For this review, take the finished solid that the model builds, in its own axes (mm). A direction names the side the tool comes from. Coordinates: 2 decimals unless noted, no trailing zeros. Loops run counter-clockwise (first coordinate to the right, second up) from the corner with the lowest first, then second, coordinate; pieces in that order, holes last. Notation, with made-up numbers: (69, 37.25) -> (117, 37.25) arc R15 ccw to (117, 52.25) -> close; hole circle Ø8 at (84, 11.5). An arc over 180 degrees is marked (long way). Answer in a Markdown table with one row per item.
from build123d import *

# Parameters (mm, degrees)
BASES_W                              = 20.16
BASES_H                              = 40
BASE_DEPTH                           = 10
SHAFTHOLES_R                         = 3
SHAFT_HOLE_DEPTH                     = 25.527666012
MOUNTINGTABS_W                       = 19
MOUNTINGTABS_H                       = 2.4
MOUNTING_TAB_DEPTH                   = 7.2
MOUNTING_HOLE_DEPTH                  = 30.986770416
BOTTOMALIGNHOLES_R                   = 0.7
BOTTOM_ALIGN_HOLE_DEPTH              = 0.5
TRIANGULAR_TAB_DEPTH                 = 0.9
MOUNTING_TAB_FEATURES_M_COPY_1_DEPTH = 30.986770416
BORDERCUTS_W                         = 20.16
BORDERCUTS_H                         = 40
BORDERCUTS_W_2                       = 19.56
BORDERCUTS_H_2                       = 39.4
BORDER_CUT_DEPTH                     = 0.5
BORDER_CUT_F_R                       = 0.75
SHELL3_OUTLINE_W                     = 17.96
SHELL3_OUTLINE_H                     = 37.8
SHELL3_OUTLINE_R                     = 3.8
SHELL3_DEPTH                         = 9.2
SHELL3_2_OUTLINE_W                   = 18.56
SHELL3_2_OUTLINE_H                   = 38.4
SHELL3_2_OUTLINE_W_2                 = 17.96
SHELL3_2_OUTLINE_H_2                 = 37.8
SHELL3_2_DEPTH                       = 8.7
SHELL3_3_DEPTH                       = 1.6
SHELL3_START                         = 1.3
SHELL3_4_DEPTH                       = 0.3
SHELL3_START_2                       = 1.6
SHELL3_5_OUTLINE_W                   = 0.2
SHELL3_5_OUTLINE_H                   = 7.2
SHELL3_5_DEPTH                       = 0.083965765
SHELL3_START_3                       = -0.1
SHELL3_6_DEPTH                       = 0.2
SKETCH2_R                            = 4.5
CUT_EXTRUDE1_DEPTH                   = 3
SKETCH3_R                            = 6
SKETCH3_R_2                          = 5.5
BOSS_EXTRUDE1_DEPTH                  = 1.25
SKETCH3_4_R                          = 5.5
BOSS_EXTRUDE2_DEPTH                  = 1.5
SKETCH3_5_R                          = 5
BOSS_EXTRUDE3_DEPTH                  = 1.75
CUT_EXTRUDE7_DEPTH                   = 31.68299855
CUT_EXTRUDE7_DEPTH_BACK              = 31.68299855
SKETCH3_6_R                          = 3
BOSS_EXTRUDE4_DEPTH                  = 1
SKETCH6_R                            = 3
CUT_EXTRUDE8_DEPTH                   = 20
SKETCH7_W                            = 12.822327898
SKETCH7_H                            = 9.709392801
CUT_EXTRUDE9_DEPTH                   = 0.5
FILLET2_R                            = 0.3


with BuildPart() as part:
    # BaseS → BASE (new body)
    with BuildSketch(Plane(origin=(0, 0, 0), x_dir=(1, 0, 0), z_dir=(0, 1, 0))):
        Rectangle(BASES_W, BASES_H)
    extrude(amount=BASE_DEPTH)

    # ShaftHoleS → SHAFT HOLE (cut, through all)
    with BuildSketch(Plane(origin=(0, 10, 0), x_dir=(1, 0, 0), z_dir=(0, 1, 0))):
        with Locations(Location((0, 10, 0), (0, 0, 270))):
            Circle(SHAFTHOLES_R)
    extrude(amount=-SHAFT_HOLE_DEPTH, mode=Mode.SUBTRACT)

    # MountingTabS → MOUNTING TAB (add)
    with BuildSketch(Plane.XY.offset(20)):
        with Locations((0, 1.2)):
            Rectangle(MOUNTINGTABS_W, MOUNTINGTABS_H)
    mounting_tab = extrude(amount=MOUNTING_TAB_DEPTH)

    # MountingHoleS → MOUNTING HOLE (cut, through all)
    with BuildSketch(Plane(origin=(0, 2.4, 0), x_dir=(1, 0, 0), z_dir=(0, 1, 0))):
        with BuildLine():
            Line((-6.25, -26.6), (-6.25, -27.2))
            Line((-6.25, -27.2), (-3.75, -27.2))
            Line((-3.75, -27.2), (-3.75, -26.6))
            ThreePointArc((-3.75, -26.6), (-5, -22.479171307), (-6.25, -26.6))
        make_face()
    mounting_hole = extrude(amount=-MOUNTING_HOLE_DEPTH, mode=Mode.SUBTRACT)

    # MH M: MOUNTING HOLE across plane
    add(mounting_hole.mirror(Plane(origin=(0, 0, 0), x_dir=(0, 0, 1), z_dir=(1, 0, 0))), mode=Mode.SUBTRACT)

    # BottomAlignHoleS → BOTTOM ALIGN HOLE (cut)
    with BuildSketch(Plane.XZ):
        with Locations(Location((0, 25.2, 0), (0, 0, 270))):
            Circle(BOTTOMALIGNHOLES_R)
    bottom_align_hole = extrude(amount=-BOTTOM_ALIGN_HOLE_DEPTH, mode=Mode.SUBTRACT)

    # TriangularTabS → TRIANGULAR TAB (add, symmetric)
    with BuildSketch(Plane(origin=(0, 0, 0), x_dir=(0, 0, -1), z_dir=(1, 0, 0))):
        Polygon((-20, 2.4), (-27.2, 2.4), (-20, 3.2), align=None)
    triangular_tab = extrude(amount=TRIANGULAR_TAB_DEPTH, both=True)

    # MOUNTING TAB FEATURES M: MOUNTING TAB, MOUNTING HOLE, BOTTOM ALIGN HOLE, TRIANGULAR TAB across plane
    add(mounting_tab.mirror(Plane.XY))
    add(mounting_hole.mirror(Plane.XY), mode=Mode.SUBTRACT)
    add(bottom_align_hole.mirror(Plane.XY), mode=Mode.SUBTRACT)
    add(triangular_tab.mirror(Plane.XY))

    # MOUNTING TAB FEATURES M copy 1 sketch → MOUNTING TAB FEATURES M copy 1 (cut, through all)
    with BuildSketch(Plane(origin=(0, 2.4, 0), x_dir=(-1, 0, 0), z_dir=(0, 1, 0))):
        with BuildLine():
            Line((-6.25, -26.6), (-6.25, -27.2))
            Line((-6.25, -27.2), (-3.75, -27.2))
            Line((-3.75, -27.2), (-3.75, -26.6))
            ThreePointArc((-3.75, -26.6), (-5, -22.479171307), (-6.25, -26.6))
        make_face()
    extrude(amount=-MOUNTING_TAB_FEATURES_M_COPY_1_DEPTH, mode=Mode.SUBTRACT)

    # BorderCutS → BORDER CUT (cut)
    with BuildSketch(Plane(origin=(0, 10, 0), x_dir=(1, 0, 0), z_dir=(0, 1, 0))):
        Rectangle(BORDERCUTS_W, BORDERCUTS_H)
        Rectangle(BORDERCUTS_W_2, BORDERCUTS_H_2, mode=Mode.SUBTRACT)
    extrude(amount=-BORDER_CUT_DEPTH, mode=Mode.SUBTRACT)

    # BORDER CUT F
    border_cut_f_edges = [part.edges().sort_by_distance(p)[0] for p in [
        (9.78, 9.75, -19.7),
        (9.78, 9.75, 19.7),
        (-9.78, 9.75, 19.7),
        (-9.78, 9.75, -19.7),
    ]]
    fillet(border_cut_f_edges, radius=BORDER_CUT_F_R)

    # Shell3: read off the stored shape, not the designer's step
    # Shell3 outline → Shell3 (cut)
    with BuildSketch(Plane(origin=(0, 0, 0), x_dir=(1, 0, 0), z_dir=(0, 1, 0))):
        Rectangle(SHELL3_OUTLINE_W, SHELL3_OUTLINE_H)
        with Locations((0, 10)):
            Circle(SHELL3_OUTLINE_R, mode=Mode.SUBTRACT)
    extrude(amount=SHELL3_DEPTH, mode=Mode.SUBTRACT)

    # Shell3 2 outline → Shell3 2 (cut)
    with BuildSketch(Plane(origin=(0, 0, 0), x_dir=(1, 0, 0), z_dir=(0, 1, 0))):
        Rectangle(SHELL3_2_OUTLINE_W, SHELL3_2_OUTLINE_H)
        Rectangle(SHELL3_2_OUTLINE_W_2, SHELL3_2_OUTLINE_H_2, mode=Mode.SUBTRACT)
    extrude(amount=SHELL3_2_DEPTH, mode=Mode.SUBTRACT)

    # Shell3 3 outline → Shell3 3 (cut)
    with BuildSketch(Plane(origin=(0, 0, 0), x_dir=(1, 0, 0), z_dir=(0, 1, 0))):
        with BuildLine():
            Line((8.7, 19.2), (8.7, 26.4))
            Line((8.7, 26.4), (7.5516331, 26.4))
            ThreePointArc((7.5516331, 26.4), (5, 21.679171307), (2.4483669, 26.4))
            Line((2.4483669, 26.4), (0.9, 26.4))
            ThreePointArc((0.9, 26.4), (0, 23.7), (-0.9, 26.4))
            Line((-0.9, 26.4), (-2.4483669, 26.4))
            ThreePointArc((-2.4483669, 26.4), (-5, 21.679171307), (-7.5516331, 26.4))
            Line((-7.5516331, 26.4), (-8.7, 26.4))
            Line((-8.7, 26.4), (-8.7, 19.2))
            Line((-8.7, 19.2), (8.7, 19.2))
        make_face()
        with BuildLine():
            Line((8.7, -26.4), (8.7, -19.2))
            Line((8.7, -19.2), (-8.7, -19.2))
            Line((-8.7, -19.2), (-8.7, -26.4))
            Line((-8.7, -26.4), (-7.5516331, -26.4))
            ThreePointArc((-7.5516331, -26.4), (-5, -21.679171307), (-2.4483669, -26.4))
            Line((-2.4483669, -26.4), (-0.9, -26.4))
            ThreePointArc((-0.9, -26.4), (0, -23.7), (0.9, -26.4))
            Line((0.9, -26.4), (2.4483669, -26.4))
            ThreePointArc((2.4483669, -26.4), (5, -21.679171307), (7.5516331, -26.4))
            Line((7.5516331, -26.4), (8.7, -26.4))
        make_face()
    extrude(amount=SHELL3_3_DEPTH, mode=Mode.SUBTRACT)

    # Shell3 4 outline → Shell3 4 (cut)
    with BuildSketch(Plane(origin=(0, 0, 0), x_dir=(1, 0, 0), z_dir=(0, 1, 0)).offset(SHELL3_START)):
        with BuildLine():
            Line((0.9, 26.4), (-0.9, 26.4))
            ThreePointArc((-0.9, 26.4), (0, 23.7), (0.9, 26.4))
        make_face()
        with BuildLine():
            ThreePointArc((0.9, -26.4), (0, -23.7), (-0.9, -26.4))
            Line((-0.9, -26.4), (0.9, -26.4))
        make_face()
    extrude(amount=SHELL3_4_DEPTH, mode=Mode.SUBTRACT)

    # Shell3 5 outline → Shell3 5 (cut)
    with BuildSketch(Plane(origin=(0, 0, 0), x_dir=(1, 0, 0), z_dir=(0, 1, 0)).offset(SHELL3_START_2)):
        with Locations((0, 22.8)):
            Rectangle(SHELL3_5_OUTLINE_W, SHELL3_5_OUTLINE_H)
        with Locations((0, -22.8)):
            Rectangle(SHELL3_5_OUTLINE_W, SHELL3_5_OUTLINE_H)
    extrude(amount=SHELL3_5_DEPTH, mode=Mode.SUBTRACT)

    # Shell3 6 outline → Shell3 6 (cut)
    with BuildSketch(Plane.YZ.offset(SHELL3_START_3)):
        Polygon((2.483965765, 19.2), (1.683965765, 26.4), (1.683965765, 19.2), align=None)
        Polygon((1.683965765, -19.2), (1.683965765, -26.4), (2.483965765, -19.2), align=None)
    extrude(amount=SHELL3_6_DEPTH, mode=Mode.SUBTRACT)

    # Sketch2 → Cut-Extrude1 (cut)
    with BuildSketch(Plane(origin=(0, 0, 0), x_dir=(-1, 0, 0), z_dir=(0, -1, 0))):
        with Locations((0, 10)):
            Circle(SKETCH2_R)
    extrude(amount=-CUT_EXTRUDE1_DEPTH, mode=Mode.SUBTRACT)

    # Sketch3 → Boss-Extrude1 (add)
    with BuildSketch(Plane(origin=(0, 10, 0), x_dir=(1, 0, 0), z_dir=(0, 1, 0))):
        with Locations(Location((0, 10, 0), (0, 0, 90))):
            Circle(SKETCH3_R)
        with Locations(Location((0, 10, 0), (0, 0, 270))):
            Circle(SKETCH3_R_2, mode=Mode.SUBTRACT)
    extrude(amount=BOSS_EXTRUDE1_DEPTH)

    # Sketch3<4> → Boss-Extrude2 (add)
    with BuildSketch(Plane(origin=(0, 10, 0), x_dir=(1, 0, 0), z_dir=(0, 1, 0))):
        with Locations(Location((0, 10, 0), (0, 0, 270))):
            Circle(SKETCH3_4_R)
    extrude(amount=BOSS_EXTRUDE2_DEPTH)

    # Sketch3<5> → Boss-Extrude3 (add)
    with BuildSketch(Plane(origin=(0, 10, 0), x_dir=(1, 0, 0), z_dir=(0, 1, 0))):
        with Locations(Location((0, 10, 0), (0, 0, 270))):
            Circle(SKETCH3_5_R)
    extrude(amount=BOSS_EXTRUDE3_DEPTH)

    # Sketch3<6> → Cut-Extrude7 (cut, two sides: drawn at the far end of the back side and taken through both)
    with BuildSketch(Plane(origin=(0, 10, 0), x_dir=(1, 0, 0), z_dir=(0, 1, 0)).offset(-CUT_EXTRUDE7_DEPTH_BACK)):
        with Locations(Location((0, 10, 0), (0, 0, 270))):
            Circle(SKETCH3_6_R)
    extrude(amount=CUT_EXTRUDE7_DEPTH + CUT_EXTRUDE7_DEPTH_BACK, mode=Mode.SUBTRACT)

    # Sketch5 → Boss-Extrude4 (add)
    with BuildSketch(Plane(origin=(0, 10, 0), x_dir=(1, 0, 0), z_dir=(0, 1, 0))):
        with BuildLine():
            Line((8, 10), (8, -15))
            Line((8, -15), (-8, -15))
            Line((-8, -15), (-8, 10))
            ThreePointArc((-8, 10), (0, 18), (8, 10))
        make_face()
    extrude(amount=BOSS_EXTRUDE4_DEPTH)

    # Sketch6 → Cut-Extrude8 (cut)
    with BuildSketch(Plane(origin=(0, 11, 0), x_dir=(1, 0, 0), z_dir=(0, 1, 0))):
        with Locations(Location((0, 10, 0), (0, 0, 270))):
            Circle(SKETCH6_R)
    extrude(amount=-CUT_EXTRUDE8_DEPTH, mode=Mode.SUBTRACT)

    # Sketch7 → Cut-Extrude9 (cut)
    with BuildSketch(Plane(origin=(0, 11, 0), x_dir=(1, 0, 0), z_dir=(0, 1, 0))):
        with Locations((0.037058751, -8.819982774)):
            Rectangle(SKETCH7_W, SKETCH7_H)
    extrude(amount=-CUT_EXTRUDE9_DEPTH, mode=Mode.SUBTRACT)

    # Fillet2
    fillet2_edges = [part.edges().sort_by_distance(p)[0] for p in [
        (0, 10, -18),
        (-8, 10, 2.5),
        (0, 10, 15),
        (8, 10, 2.5),
        (0, 11, -18),
        (-8, 11, 2.5),
        (0, 11, 15),
        (8, 11, 2.5),
    ]]
    fillet(fillet2_edges, radius=FILLET2_R)


solid = part.part
Item 1: Take a section at C-C, the plane z = 23. Count the separate pieces of the cut face and the enclosed holes in it, and give its area (3 significant figures).
Worked answers:
| item | result |
|---|---|
| separate pieces | 3 |
| enclosed holes | 0 |
| area | 20.8 mm² |
Item 2: The part is to be moulded in two halves that separate along Z. For faces 3 (the flat face through (8, 1, -27.2)), 4 (the flat face through (-3.5, 1.6, 21.9)), 5 (the flat face through (-8, 1, -26.4)), 6 (the flat face through (8, 1, 27.2)), say which applies: +Z half, -Z half, draft (parallel to the pull), parting line (faces both ways), or undercut.
Worked answers:
| item | result |
|---|---|
| face 3 | -Z half |
| face 4 | undercut |
| face 5 | undercut |
| face 6 | +Z half |
Item 3: Take a section at A-A, the plane y = 5.75. State the section outline as (x, z) points, and give its area (3 significant figures).
Worked answers:
| item | result |
|---|---|
| outline | (-10.08, -20) -> (10.08, -20) -> (10.08, 20) -> (-10.08, 20) -> close; circle Ø7.6 at (0, -10); hole (-9.28, -19.2) -> (9.28, -19.2) -> (9.28, 19.2) -> (-9.28, 19.2) -> close; hole circle Ø6 at (0, -10) |
| area | 111 mm² |
Item 4: For faces 1 (the cylindrical face through (-4.92, 1.22, -22.48)), 2 (the flat face through (0, 5, 19.2)), list the 3-axis set-ups (+Z, -Z, +X, -X, +Y, -Y) from which the entire face can be reached by the end or side of a thin tool; tool diameter is ignored.
Worked answers:
| item | result |
|---|---|
| face 1 | +Y, -Y |
| face 2 | -Y |
Item 5: Take a section at D-D, the plane z = 10. State the section outline as (x, y) points.
Worked answers:
| item | result |
|---|---|
| outline | (-10.08, 0) -> (-9.28, 0) -> (-9.28, 8.7) -> (-8.98, 8.7) -> (-8.98, 9.2) -> (8.98, 9.2) -> (8.98, 8.7) -> (9.28, 8.7) -> (9.28, 0) -> (10.08, 0) -> (10.08, 9.5) -> (9.78, 9.5) -> (9.78, 10) -> (8.3, 10) arc R0.3 cw to (8, 10.3) -> (8, 10.7) arc R0.3 ccw to (7.7, 11) -> (6.45, 11) -> (6.45, 10.5) -> (-6.37, 10.5) -> (-6.37, 11) -> (-7.7, 11) arc R0.3 ccw to (-8, 10.7) -> (-8, 10.3) arc R0.3 cw to (-8.3, 10) -> (-9.78, 10) -> (-9.78, 9.5) -> (-10.08, 9.5) -> close |
Item 6: Take a section at B-B, the plane z = 16. State the section outline as (x, y) points, and give its area (3 significant figures).
Worked answers:
| item | result |
|---|---|
| outline | (-10.08, 0) -> (-9.28, 0) -> (-9.28, 8.7) -> (-8.98, 8.7) -> (-8.98, 9.2) -> (8.98, 9.2) -> (8.98, 8.7) -> (9.28, 8.7) -> (9.28, 0) -> (10.08, 0) -> (10.08, 9.5) -> (9.78, 9.5) -> (9.78, 10) -> (-9.78, 10) -> (-9.78, 9.5) -> (-10.08, 9.5) -> close |
| area | 30.8 mm² |
Item 7: For L1, parallel to Z at x = 0, y = 3.5; L2, parallel to X at y = 2, z = 24.5; L3, parallel to X at y = 0.5, z = 18, list the stretches that pass through material, from the lowest coordinate up.
Worked answers:
| item | result |
|---|---|
| L1 | -20 to -19.2, -13.8 to -13, -7 to -6.2, 19.2 to 20 |
| L2 | -9.5 to -7.24, -2.76 to 2.76, 7.24 to 9.5 |
| L3 | -10.08 to -9.28, 9.28 to 10.08 |
Item 8: Insertion check: pin 1 (0.6 mm diameter, centred on x = 3, y = 11, fed in from -Z); pin 2 (0.6 mm diameter, centred on y = 3, z = -23, fed in from +X); pin 3 (9.5 mm diameter, centred on x = -0.5, z = 0.5, fed in from -Y). Each pin has a flat end and moves straight along its axis. Give the tip position at first contact, or say it passes through.
Worked answers:
| item | result |
|---|---|
| pin 1 | z = -17.48 |
| pin 2 | x = 0.9 |
| pin 3 | y = 9.2 |
